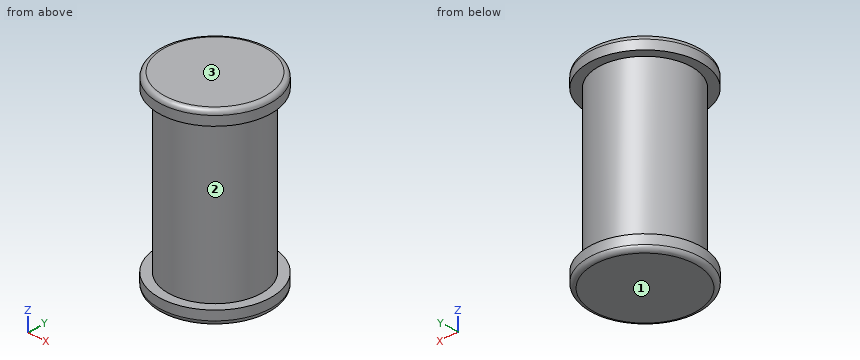
from build123d import *

# Parameters (mm, degrees)
SKETCH_1_R        = 10
EXTRUDE_1_DEPTH   = 40
EXTRUDE_START     = -3
SKETCH_3_R        = 12
SKETCH_3_R_2      = 10
EXTRUDE_1_2_DEPTH = 3
SKETCH_4_R        = 12
SKETCH_4_R_2      = 10
EXTRUDE_2_DEPTH   = 3
FILLET_4_R        = 1


with BuildPart() as part:
    # 草图1 → Extrude 1 (new body)
    with BuildSketch(Plane.XY):
        Circle(SKETCH_1_R)
    extrude(amount=EXTRUDE_1_DEPTH)

    # 草图3 → Extrude 1 2 (add)
    with BuildSketch(Plane.XY.offset(40).offset(EXTRUDE_START)):
        Circle(SKETCH_3_R)
        Circle(SKETCH_3_R_2, mode=Mode.SUBTRACT)
    extrude(amount=EXTRUDE_1_2_DEPTH)

    # 草图4 → 拉伸-薄壁2 (add)
    with BuildSketch(Plane(origin=(0, 0, 0), x_dir=(-1, 0, 0), z_dir=(0, 0, -1))):
        Circle(SKETCH_4_R)
        Circle(SKETCH_4_R_2, mode=Mode.SUBTRACT)
    extrude(amount=-EXTRUDE_2_DEPTH)

    # 圆角4
    fillet_4_edges = [part.edges().sort_by_distance(p)[0] for p in [
        (12, 0, 0),
        (-12, 0, 40),
    ]]
    fillet(fillet_4_edges, radius=FILLET_4_R)


solid = part.part
Work out the finished part from the listing and answer in its coordinate system (mm). Face numbers are marked on the shaded views. Give positions to 0.01 mm unless a question says otherwise; leave off trailing zeros. Write each loop counter-clockwise with the first axis right and the second up, starting at its lowest first coordinate (ties: lowest second). Pieces come first, ordered by that corner, then holes. Notation, with made-up numbers: M -18,-34.75 L 29,-34.75 A35 ccw 29,4.25 Z; hole C -19.5,31.5 d10. An arc over 180 degrees is marked long. Answer as CSV lines item,"result".
Q1. The mould has two halves that part along Z. Classify the marked faces 1, 2 and 3: +Z half, -Z half, draft (parallel to the pull), parting line (faces both ways), or undercut.
A:
face 1,"-Z half"
face 2,"undercut"
face 3,"+Z half"
Q2. A cutting plane is placed at C-C on z = 24.5. Write down the section's boundary in (x, y).
A:
outline,"C 0,0 d20"
Q3. Find the intervals of material crossed by probe 1 along Z at (x, y) = (10.25, -0.25); probe 2 along Y at (x, z) = (-5, 34); probe 3 along X at (y, z) = (-4.75, 4), in increasing order. Write a range as [from, to].
A:
probe 1,"z = [0, 3], [37, 40]"
probe 2,"y = [-8.66, 8.66]"
probe 3,"x = [-8.8, 8.8]"
Q4. A cutting plane is placed at A-A on x = 0. Write down the section's boundary in (y, z), plus the area to 3 significant figures.
A:
outline,"M -12,1 A1 ccw -11,0 L 11,0 A1 ccw 12,1 L 12,3 L 10,3 L 10,37 L 12,37 L 12,39 A1 ccw 11,40 L -11,40 A1 ccw -12,39 L -12,37 L -10,37 L -10,3 L -12,3 Z"
area,"823 mm²"
Q5. Given P1, Ø10, axis at x = 0, z = 6.5, coming from the +Y side; P2, Ø6, axis at y = 4.5, z = 33, coming from the -X side; P3, Ø4, axis at x = -2, z = 32.5, coming from the +Y side; P4, Ø3, axis at y = 5.5, z = 19.5, coming from the -X side, each flat-ended and moving along its own axis, determine where each tip first touches the part or whether it passes through.
A:
P1,"stops at y = 12"
P2,"stops at x = -9.89"
P3,"stops at y = 10"
P4,"stops at x = -9.17"
